from build123d import *

# Parameters (mm, degrees)
F1_DEPTH = 40.2336
F0_R     = 10.16
F2_DEPTH = 15.7734
F3_R     = 3.302


with BuildPart() as f1:
    # F0 (on Top) → F1 (new body)
    with BuildSketch(Plane.XY):
        with BuildLine():
            ThreePointArc((-46.787253, -28.063018), (-30.144883, -18.202414), (-23.597202, 0))
            ThreePointArc((-23.597202, 0), (-30.144883, 18.202414), (-46.787253, 28.063018))
            ThreePointArc((-46.787253, 28.063018), (-80.747202, 0), (-46.787253, -28.063018))
        make_face()
        with BuildLine():
            ThreePointArc((-38.724437, -4.826), (-66.459702, 0), (-38.724437, 4.826))
            Line((-38.724437, 4.826), (-33.642902, 4.826))
            Line((-33.642902, 4.826), (-33.642902, -4.826))
            Line((-33.642902, -4.826), (-38.724437, -4.826))
        make_face(mode=Mode.SUBTRACT)
    extrude(amount=F1_DEPTH)

    # F0 (on Top) → F2 (join)
    with BuildSketch(Plane.XY):
        with BuildLine():
            ThreePointArc((-46.787253, -28.063018), (-30.144883, -18.202414), (-23.597202, 0))
            ThreePointArc((-23.597202, 0), (-30.144883, 18.202414), (-46.787253, 28.063018))
            ThreePointArc((-46.787253, 28.063018), (-80.747202, 0), (-46.787253, -28.063018))
        make_face()
        with BuildLine():
            ThreePointArc((-38.724437, -4.826), (-66.459702, 0), (-38.724437, 4.826))
            Line((-38.724437, 4.826), (-33.642902, 4.826))
            Line((-33.642902, 4.826), (-33.642902, -4.826))
            Line((-33.642902, -4.826), (-38.724437, -4.826))
        make_face(mode=Mode.SUBTRACT)
        with BuildLine():
            ThreePointArc((-46.787253, 28.063018), (-30.144883, 18.202414), (-23.597202, 0))
            ThreePointArc((-23.597202, 0), (-30.144883, -18.202414), (-46.787253, -28.063018))
            Line((-46.787253, -28.063018), (10.103749, -17.146333))
            ThreePointArc((10.103749, -17.146333), (20.852798, 0), (10.103749, 17.146333))
            Line((10.103749, 17.146333), (-46.787253, 28.063018))
        make_face()
        with Locations((1.802798, 0)):
            Circle(F0_R, mode=Mode.SUBTRACT)
    extrude(amount=F2_DEPTH)

    # F3
    f3_edges = [f1.edges().sort_by_distance(p)[0] for p in [
        (-57.55715, 28.063018, 40.2336),
    ]]
    fillet(f3_edges, radius=F3_R)


solid = f1.part
Design review of the part built by this model. Coordinates are the model's own, in mm. A direction names the side the tool comes from. Round coordinates to 2 decimals unless told otherwise and drop trailing zeros.
Item 1: Consider section A-A on z = 13. Count the separate pieces of the cut face and the enclosed holes in it, and give its area (3 significant figures).
Item 2: Wall thickness on L1, parallel to X at y = 0, z = 17; L2, parallel to X at y = 6, z = 4.5; L3, parallel to X at y = 7, z = 4.5: over which ranges is each line inside the solid? List them lowest first.
Item 3: For faces 4 (the flat face through (-36, -4.826, 20)), 5 (the flat face through (-31, 0, 0)), list the 3-axis set-ups (+Z, -Z, +X, -X, +Y, -Y) from which the entire face can be reached by the end or side of a thin tool; tool diameter is ignored.
Item 4: Draft analysis for pull direction X (two halves, no side actions). For faces 1 (the flat face through (-36, 4.826, 20)), 2 (the flat face through (-13, 0, 15.773)), 3 (the flat face through (-18.74, -22.68, 7.78)), state which applies: released by +X, released by -X, zero draft, split by the parting line, or undercut.
Item 5: For pin 1 Ø6 at (y, z) = (22, 31) entering from +X; pin 2 Ø3 at (x, y) = (-8.5, -10) entering from +Z; pin 3 Ø1.5 at (x, y) = (-48.5, -14.5) entering from -Z; pin 4 Ø10 at (x, z) = (-9.5, 11) entering from +Y, all flat-tipped, find the tip position at first contact; note any pin that passes through.
Check values:
1. separate pieces: 1
1. enclosed holes: 2
1. area: 3,420 mm2
2. L1: x = -80.75 to -66.46, -33.64 to -23.6
2. L2: x = -80.11 to -65.14, -39.21 to -6.4, 10 to 19.88
2. L3: x = -79.88 to -64.63, -39.72 to -5.56, 9.17 to 19.52
3. face 4: +Z, -Z
3. face 5: -Z, +X, -X, +Y, -Y
4. face 1: undercut
4. face 2: zero draft
4. face 3: released by +X
5. pin 1: stops at x = -30.83
5. pin 2: stops at z = 15.77
5. pin 3: stops at z = 0
5. pin 4: stops at y = 21.87
